from build123d import *

# Parameters (mm, degrees)
SKETCH1_R          = 19.05
SKETCH1_R_2        = 15.875
CUT_EXTRUDE1_START = -7.9375
CUT_EXTRUDE1_DEPTH = 7.9375


with BuildPart() as part:
    # Sweep1: sweep along a path in Sketch2
    with BuildLine(Plane(origin=(0, 0, 0), x_dir=(0, 0, -1), z_dir=(1, 0, 0))) as sweep1_path:
        Line((0, 0), (38.1, 0))
        ThreePointArc((38.1, 0), (60.550640303, 9.299359697), (69.85, 31.75))
    # Sketch1 → Sweep1 (sweep)
    with BuildSketch(Plane.XY):
        Circle(SKETCH1_R)
        Circle(SKETCH1_R_2, mode=Mode.SUBTRACT)
    sweep(path=sweep1_path.line)

    # Sketch3 → Cut-Extrude1 (cut)
    with BuildSketch(Plane.XY.offset(-25.4).offset(CUT_EXTRUDE1_START)):
        with BuildLine():
            Line((-19.05, 0), (-15.875, 0))
            ThreePointArc((-15.875, 0), (0, 15.875), (15.875, 0))
            Line((15.875, 0), (19.05, 0))
            ThreePointArc((19.05, 0), (0, 19.05), (-19.05, 0))
        make_face()
    extrude(amount=CUT_EXTRUDE1_DEPTH, mode=Mode.SUBTRACT)


solid = part.part
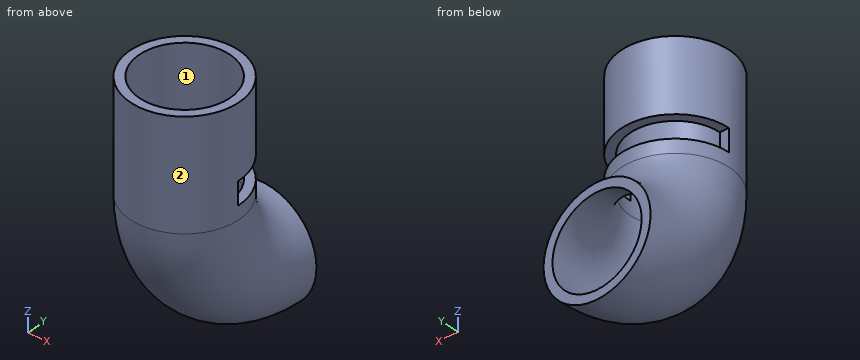
Design review of the part built by this model. Coordinates are the model's own, in mm. Face numbers are marked on the shaded views. Round coordinates to 2 decimals unless told otherwise and drop trailing zeros. Write each loop counter-clockwise with the first axis right and the second up, starting at its lowest first coordinate (ties: lowest second). Pieces come first, ordered by that corner, then holes. Notation, with made-up numbers: M -34,33.25 L -3,33.25 A35 ccw -3,65.25 Z; hole C 43,83.25 d11. An arc over 180 degrees is marked long. One line per item, written item: value. Start each with the question number.
1. Take a section at A-A on x = 10. State the section outline as (y, z) points.
2. To check wall thickness, follow probe 1 along Y at (x, z) = (0, -15) (3 decimals); probe 2 along Z at (x, y) = (4, 17); probe 3 along X at (y, z) = (0, -59). State the ranges of each line that lie inside material, in increasing order. Write a range as from..to.
3. Clearance check with flat-ended pins moving along their axes: P1, Ø1.5, axis at x = -9, z = -75, coming from the +Y side; P2, Ø21, axis at x = 0.5, y = 8.5, coming from the +Z side; P3, Ø2, axis at y = 9.5, z = -46, coming from the +X side; P4, Ø15, axis at x = 9, y = 11.5, coming from the -Z side. State where each tip first meets the part, or that it passes through.
4. Take a section at D-D on z = -31. State the section outline as (x, y) points (3 decimals), then the cut area to 3 significant figures.
5. Take a section at B-B on z = -16. State the section outline as (x, y) points (3 decimals).
6. Draft analysis for pull direction Y (two halves, no side actions). For the marked faces 1 and 2, state which applies: pulls with the +Y half, pulls with the -Y half, needs draft (parallel to the pull), parting line crosses it, or undercut.
7. Take a section at C-C on y = 8. State how many separate pieces and enclosed holes the cut face has, then the cut area to 3 significant figures.
Computed:
1. outline: M -16.21,-38.1 A47.96 ccw 31.75,-86.06 L 31.75,-82.18 A44.08 cw -12.33,-38.1 L -12.33,0 L -16.21,0 Z; M 12.33,-38.1 A19.42 ccw 31.75,-57.52 L 31.75,-53.64 A15.54 cw 16.21,-38.1 L 16.21,-33.34 L 12.33,-33.34 Z; M 12.33,-25.4 L 16.21,-25.4 L 16.21,0 L 12.33,0 Z
2. probe 1: y = -19.05..-15.875, 15.875..19.05
2. probe 2: z = -86.27..-82.84, -45.24..-33.34, -25.4..0
2. probe 3: x = -17.99..-14.59, 14.59..17.99
3. P1: stops at y = 7.79
3. P2: stops at z = 0
3. P3: stops at x = 17.66
3. P4: stops at z = -86.3
4. outline: M -19.05,0 A19.05 ccw 19.05,0 L 15.875,0 A15.875 cw -15.875,0 Z
4. area: 174 mm²
5. outline: C 0,0 d38.1; hole C 0,0 d31.75
6. face 1: undercut
6. face 2: parting line crosses it
7. separate pieces: 3
7. enclosed holes: 0
7. area: 571 mm²
